The listing builds one solid part. Answer for the finished solid, in the listing's coordinates (mm). Give positions to 0.01 mm unless a question says otherwise; leave off trailing zeros. Loops run counter-clockwise (first coordinate to the right, second up) from the corner with the lowest first, then second, coordinate; pieces in that order, holes last. Notation, with made-up numbers: M 77.25,70.5 L 87.25,70.5 A20 ccw 87.25,97.5 Z; hole C 42.5,-23.75 d11. An arc over 180 degrees is marked long. One line per item, written item: value. Start each with the question number.
Q1. A cutting plane is placed at A-A, the plane z = 0.9. State how many separate pieces and enclosed holes the cut face has, and give its area (3 significant figures).
Q2. Flat-ended cylindrical pins translate along their axes: pin 1 (0.9 mm diameter, centred on y = -1.5, z = 1, fed in from +X); pin 2 (0.9 mm diameter, centred on y = 84, z = 2, fed in from -X); pin 3 (0.9 mm diameter, centred on x = -135, z = 1.5, fed in from -Y). Find the tip coordinate at first contact, or state that the pin passes through.
Q3. A cutting plane is placed at B-B, the plane x = 63.5. Determine the outline of the cut face in (y, z).
Q4. Consider L1, parallel to X at y = 59, z = 1.15; L2, parallel to X at y = 15, z = 0.2; L3, parallel to Y at x = -68, z = 2.85. Determine where each line is inside the solid, lowest interval first.
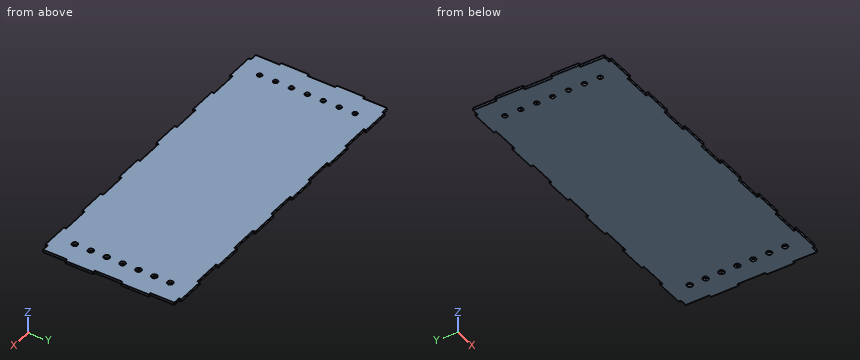
from build123d import *

# Parameters (mm, degrees)
BOSS_EXTRUDE1_DEPTH = 3
SKETCH1_R           = 3
SKETCH1_R_2         = 3.5
CUT_EXTRUDE1_DEPTH  = 222.674310645


with BuildPart() as part:
    # Model → Boss-Extrude1 (new body)
    with BuildSketch(Plane.XY):
        Polygon((192.5, 85.5), (157.5, 85.5), (157.5, 82.5), (122.5, 82.5), (122.5, 85.5), (87.5, 85.5), (87.5, 82.5), (52.5, 82.5), (52.5, 85.5), (17.5, 85.5), (17.5, 82.5), (-17.5, 82.5), (-17.5, 85.5), (-52.5, 85.5), (-52.5, 82.5), (-87.5, 82.5), (-87.5, 85.5), (-122.5, 85.5), (-122.5, 82.5), (-157.5, 82.5), (-157.5, 85.5), (-192.5, 85.5), (-192.5, 82.5), (-201.5, 82.5), (-201.5, 52.5), (-204.5, 52.5), (-204.5, 17.5), (-201.5, 17.5), (-201.5, -17.5), (-204.5, -17.5), (-204.5, -52.5), (-201.5, -52.5), (-201.5, -82.5), (-192.5, -82.5), (-192.5, -85.5), (-157.5, -85.5), (-157.5, -82.5), (-122.5, -82.5), (-122.5, -85.5), (-87.5, -85.5), (-87.5, -82.5), (-52.5, -82.5), (-52.5, -85.5), (-17.5, -85.5), (-17.5, -82.5), (17.5, -82.5), (17.5, -85.5), (52.5, -85.5), (52.5, -82.5), (87.5, -82.5), (87.5, -85.5), (122.5, -85.5), (122.5, -82.5), (157.5, -82.5), (157.5, -85.5), (192.5, -85.5), (192.5, -82.5), (201.5, -82.5), (201.5, -52.5), (204.5, -52.5), (204.5, -17.5), (201.5, -17.5), (201.5, 17.5), (204.5, 17.5), (204.5, 52.5), (201.5, 52.5), (201.5, 82.5), (192.5, 82.5), align=None)
    extrude(amount=BOSS_EXTRUDE1_DEPTH)

    # Sketch1 → Cut-Extrude1 (cut, through all)
    with BuildSketch(Plane.XY.offset(3)):
        with Locations((-175, 0)):
            Circle(SKETCH1_R)
        with Locations((175, 0)):
            Circle(SKETCH1_R_2)
        with Locations((-175, 20)):
            Circle(SKETCH1_R)
        with Locations((175, 20)):
            Circle(SKETCH1_R_2)
        with Locations((-175, 40)):
            Circle(SKETCH1_R)
        with Locations((175, 40)):
            Circle(SKETCH1_R_2)
        with Locations((-175, 60)):
            Circle(SKETCH1_R)
        with Locations((175, 60)):
            Circle(SKETCH1_R_2)
        with Locations((-175, -20)):
            Circle(SKETCH1_R)
        with Locations((175, -20)):
            Circle(SKETCH1_R_2)
        with Locations((-175, -40)):
            Circle(SKETCH1_R)
        with Locations((175, -40)):
            Circle(SKETCH1_R_2)
        with Locations((-175, -60)):
            Circle(SKETCH1_R)
        with Locations((175, -60)):
            Circle(SKETCH1_R_2)
    extrude(amount=-CUT_EXTRUDE1_DEPTH, mode=Mode.SUBTRACT)


solid = part.part
Answer block:
1. separate pieces: 1
1. enclosed holes: 14
1. area: 67,700 mm^2
2. pin 1: x = 201.5
2. pin 2: x = -192.5
2. pin 3: y = -82.5
3. outline: M -82.5,0 L 82.5,0 L 82.5,3 L -82.5,3 Z
4. L1: -201.5 to -177.83, -172.17 to 171.65, 178.35 to 201.5
4. L2: -201.5 to 201.5
4. L3: -82.5 to 82.5
